Read the model definition and answer for the solid it produces. Units are mm, in the model's axes. Face numbers are marked on the shaded views. Give positions to 0.01 mm unless a question says otherwise; leave off trailing zeros. Order: outer loops, then holes, each group sorted by start corner. A loop starts at its lowest first (then second) coordinate and runs counter-clockwise, first axis right, second up.
Item 1: A cutting plane is placed at B-B (y = 73). Write down the section's boundary in (x, z), plus the area to 3 significant figures.
Item 2: A cutting plane is placed at A-A (z = 0). Write down the section's boundary in (x, y).
Item 3: A cutting plane is placed at C-C (x = 12). Write down the section's boundary in (y, z).
Item 4: The mould has two halves that part along Z. Classify the marked faces 1, 2 and 3: +Z half, -Z half, draft (parallel to the pull), parting line (faces both ways), or undercut.
Item 5: Find the intervals of material crossed by line 1 along Y through (x, z) = (92, 1); line 2 along X through (y, z) = (72, 2.5); line 3 along Y through (x, z) = (11.5, -0.5), in increasing order.
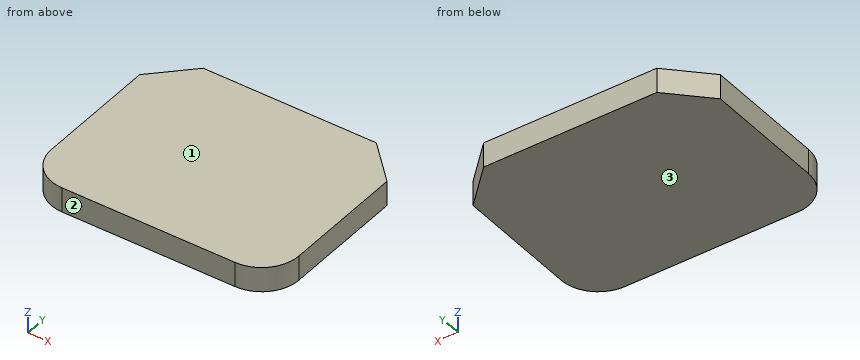
Autodesk Inventor part; units mm, degrees
ref_plane "YZ Plane" through (0, 0, 0) normal (1, 0, 0) x (0, 1, 0)
ref_plane "XZ Plane" through (0, 0, 0) normal (0, 1, 0) x (-1, 0, 0)
ref_plane "XY Plane" through (0, 0, 0) normal (0, 0, 1) x (1, 0, 0)
sketch "Sketch1" plane through (0, 0, 0) normal (0, 0, 1) x (1, 0, 0)
  line L0 (0, 0) -> (100, 0)
  line L1 (100, 0) -> (100, 80)
  line L2 (100, 80) -> (0, 80)
  line L3 (0, 80) -> (0, 0)
  circle A0 centre (15, 15) radius 5
  circle A1 centre (85, 15) radius 5
  circle A2 centre (85, 65) radius 5
  circle A3 centre (15, 65) radius 5
  dimension "d0" = 100
  dimension "d1" = 80
  dimension "d12" = 10
  dimension "d13" = 10
  dimension "d14" = 10
  dimension "d15" = 10
  dimension "d17" = 15
  dimension "d18" = 15
  dimension "d19" = 15
  dimension "d20" = 15
  dimension "d21" = 15
  dimension "d22" = 15
  dimension "d23" = 15
  dimension "d24" = 15
extrude "Extrusion1" add sketch "Sketch1" along normal mid plane 10 contours L3 L2 L1 L0 | A0 | A1 | A2 | A3
sketch "Sketch2" plane through (0, 0, 5) normal (0, 0, 1) x (1, 0, 0)
  point P0 (0, 0)
chamfer "Chamfer1" distance 15 angle 45 1 edges at (100, 80, 0)
chamfer "Chamfer2" distance 15 angle 45 1 edges at (0, 80, 0)
fillet "Fillet1" radius 15 1 edges at (100, 0, 0)
fillet "Fillet2" radius 15 1 edges at (0, 0, 0)
sketch "Sketch3" plane through (0, 0, 5) normal (0, 0, 1) x (1, 0, 0)
  point P0 (0, 0)
Response values:
1. outline: (8, -5) - (92, -5) - (92, 5) - (8, 5) - close
1. area: 840 mm2
2. outline: (0, 15) arc R15 ccw to (15, 0) - (85, 0) arc R15 ccw to (100, 15) - (100, 65) - (85, 80) - (15, 80) - (0, 65) - close
3. outline: (0.3, -5) - (77, -5) - (77, 5) - (0.3, 5) - close
4. face 1: +Z half
4. face 2: draft
4. face 3: -Z half
5. line 1: y = 1.73 to 73
5. line 2: x = 7 to 93
5. line 3: y = 0.41 to 76.5
